```python
from build123d import *

# Parameters (mm, degrees)
F0_R     = 1.575
F0_W     = 14.697724
F0_H     = 16.5
F0_W_2   = 2.5
F0_H_2   = 23.769202
F1_DEPTH = 2


with BuildPart() as f1:
    # F0 (on Top) → F1 (new body)
    with BuildSketch(Plane.XY):
        with BuildLine():
            ThreePointArc((-18, -15.999481), (-17.414214, -17.413694), (-16, -17.999481))
            Line((-16, -17.999481), (-7.348862, -17.999481))
            Line((-7.348862, -17.999481), (7.348862, -17.999481))
            Line((7.348862, -17.999481), (16, -17.999481))
            ThreePointArc((16, -17.999481), (17.414214, -17.413694), (18, -15.999481))
            Line((18, -15.999481), (18, -11.884601))
            Line((18, -11.884601), (18, 11.884601))
            Line((18, 11.884601), (18, 15.999481))
            ThreePointArc((18, 15.999481), (17.414214, 17.413694), (16, 17.999481))
            Line((16, 17.999481), (-16, 17.999481))
            ThreePointArc((-16, 17.999481), (-17.414214, 17.413694), (-18, 15.999481))
            Line((-18, 15.999481), (-18, 11.884601))
            Line((-18, 11.884601), (-18, -11.884601))
            Line((-18, -11.884601), (-18, -15.999481))
        make_face()
        with Locations((-15.025322, -15.249588)):
            Circle(F0_R, mode=Mode.SUBTRACT)
        with Locations((15.473853, -15.025322)):
            Circle(F0_R, mode=Mode.SUBTRACT)
        with Locations((-15.249588, 15.249588)):
            Circle(F0_R, mode=Mode.SUBTRACT)
        with Locations((15.249588, 15.473853)):
            Circle(F0_R, mode=Mode.SUBTRACT)
        with Locations((0, -26.249481)):
            Rectangle(F0_W, F0_H)
        with Locations((-19.25, 0)):
            Rectangle(F0_W_2, F0_H_2)
        with Locations((19.25, 0)):
            Rectangle(F0_W_2, F0_H_2)
    extrude(amount=F1_DEPTH)


solid = f1.part
```
Can you work these out from the model? Positions are in its coordinate system, mm. A direction names the side the tool comes from. Give positions to 0.01 mm unless a question says otherwise; leave off trailing zeros. Write each loop counter-clockwise with the first axis right and the second up, starting at its lowest first coordinate (ties: lowest second). Pieces come first, ordered by that corner, then holes. Notation, with made-up numbers: (-29.5, 41) - (-24.5, 41) arc R13 ccw to (-24.5, 58) - close; hole circle Ø10 at (-7, 49.25). An arc over 180 degrees is marked (long way). Write item = value, one per line. Start each with the question number.
1. Thinking about a two-plate mould opening in Y: for faces 1 (the face through (-17.4, 17.43, 0.99)), 2 (the face through (15.269, -13.464, 0.986)), 3 (the face through (12, -17.999, 1)), which applies, released by +Y, released by -Y, zero draft, split by the parting line, or undercut?
2. For pin 1 (0.6 mm diameter, centred on y = -22.5, z = 1, fed in from -X); pin 2 (1 mm diameter, centred on x = -19.5, z = 1.5, fed in from +Y); pin 3 (0.6 mm diameter, centred on x = -10.5, z = 0.5, fed in from -Y), each with a flat end and sliding along its axis, tell me the tip position at first contact or that it passes through.
3. Imagine slicing it at C-C (x = -9). Please give me the cut outline in (y, z).
4. Please list where these lines run through material, in increasing order: line 1 (Y direction, x = -14.5, z = 1.75); line 2 (Y direction, x = 15.5, z = 1.65); line 3 (X direction, y = -19, z = 0.7).
5. Imagine slicing it at A-A (z = 0.4). Please give me the cut outline in (x, y) (3 decimals).
6. Imagine slicing it at B-B (y = -22.5). Please give me the cut outline in (x, z), and give its area (3 significant figures).
7. On a 3-axis mill with a long thin cutter (end or side, diameter ignored), from which of +Z, -Z, +X, -X, +Y, -Y can I reach the whole of each face in a straight line? I mean faces 4 (the face through (18, -14, 1)), 5 (the face through (19, 11.885, 1)), 6 (the face through (-7.349, -26, 1)), 7 (the face through (-19, 11.885, 1)). Say none if no direction works.
Worked answers:
q1.face_1 = released by +Y
q1.face_2 = undercut
q1.face_3 = released by -Y
q2.pin_1 = -7.35
q2.pin_2 = 11.88
q2.pin_3 = -18
q3.outline = (-18, 0) - (18, 0) - (18, 2) - (-18, 2) - close
q4.line_1 = -18 to -16.73, -13.76 to 13.86, 16.63 to 18
q4.line_2 = -18 to -16.6, -13.45 to 13.92, 17.03 to 18
q4.line_3 = -7.35 to 7.35
q5.outline = (-20.5, -11.885) - (-18, -11.885) - (-18, -15.999) arc R2 ccw to (-16, -17.999) - (-7.349, -17.999) - (-7.349, -34.499) - (7.349, -34.499) - (7.349, -17.999) - (16, -17.999) arc R2 ccw to (18, -15.999) - (18, -11.885) - (20.5, -11.885) - (20.5, 11.885) - (18, 11.885) - (18, 15.999) arc R2 ccw to (16, 17.999) - (-16, 17.999) arc R2 ccw to (-18, 15.999) - (-18, 11.885) - (-20.5, 11.885) - close; hole circle Ø3.15 at (-15.25, 15.25); hole circle Ø3.15 at (-15.025, -15.25); hole circle Ø3.15 at (15.25, 15.474); hole circle Ø3.15 at (15.474, -15.025)
q6.outline = (-7.35, 0) - (7.35, 0) - (7.35, 2) - (-7.35, 2) - close
q6.area = 29.4 mm2
q7.face_4 = +Z, -Z, +X, -Y
q7.face_5 = +Z, -Z, +X, +Y
q7.face_6 = +Z, -Z, -X, -Y
q7.face_7 = +Z, -Z, -X, +Y
